Design review of the part shown in the three views and the two pictorial views. Dimensions are in mm from the part's minimum x, y and z. Give positions to 0.01 mm unless a question says otherwise; leave off trailing zeros. Write each loop counter-clockwise with the first axis right and the second up, starting at its lowest first coordinate (ties: lowest second). Pieces come first, ordered by that corner, then holes. Notation, with made-up numbers: M -11,12 L 19,12 A14 cw 19,26 Z; hole C 35.25,35.25 d3. An arc over 180 degrees is marked long. Use one line per item in the form item = value. Start each with the question number.
Q1. Consider section C-C on y = 2. Write out the cut boundary in (x, z).
Q2. Consider section B-B on z = 10.5. Write out the cut boundary in (x, y), and give its area (3 significant figures).
Q3. For probe 1 along X at (y, z) = (5.5, 47.5); probe 2 along Y at (x, z) = (33.5, 42.5) (1 decimal); probe 3 along Y at (x, z) = (19, 4), list the stretches that pass through material, from the lowest coordinate up. Write a range as [from, to].
Q4. Clearance check with flat-ended pins moving along their axes: pin 1 Ø6 at (x, z) = (18, 17.5) entering from +Y; pin 2 Ø1 at (x, y) = (12.5, 6) entering from +Z; pin 3 Ø1.1 at (x, y) = (1, 5) entering from -Z. State where each tip first meets the part, or that it passes through.
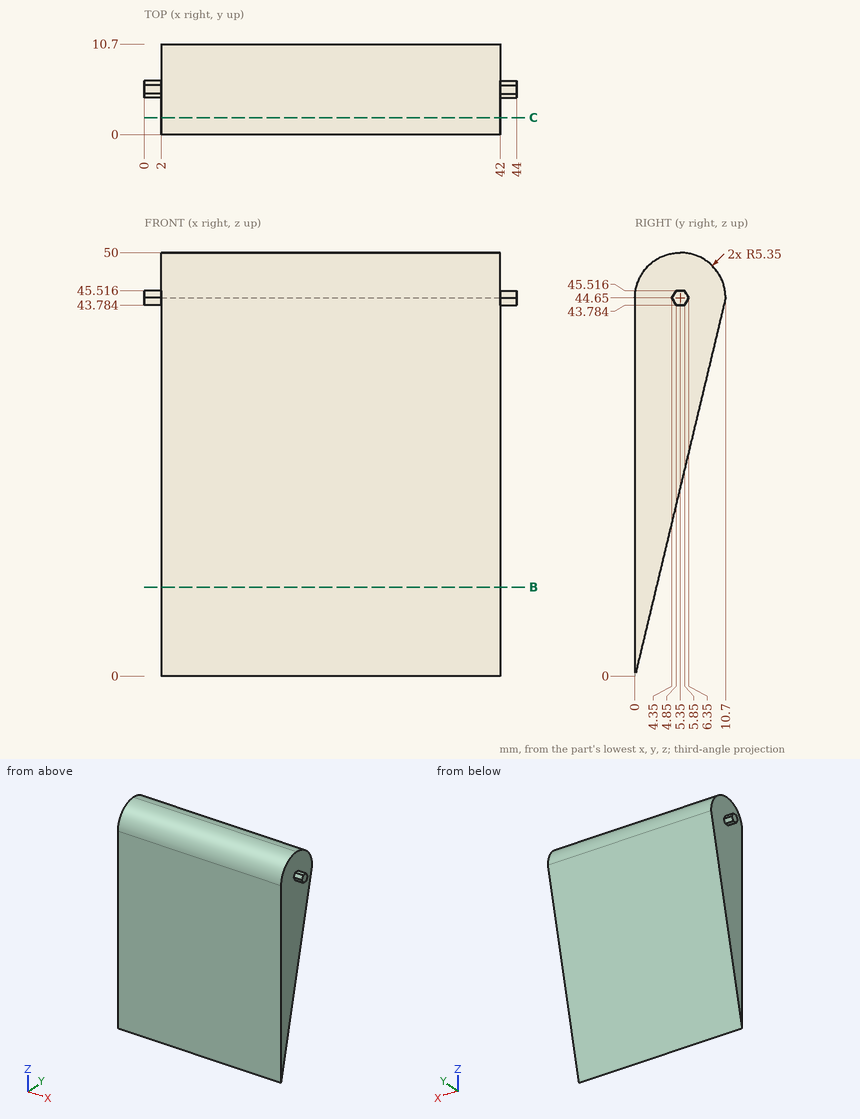
Working result:
q1.outline = M 2,8.35 L 42,8.35 L 42,48.82 L 2,48.82 Z
q2.outline = M 2,0 L 42,0 L 42,2.52 L 2,2.52 Z
q2.area = 101 mm²
q3.probe_1 = [2, 42]
q3.probe_2 = [0, 10.2]
q3.probe_3 = [0, 0.96]
q4.pin_1 = 4.91
q4.pin_2 = 50
q4.pin_3 = 43.78
